```python
from build123d import *

# Parameters (mm, degrees)
SKETCH1_R           = 27.5
BOSS_EXTRUDE1_DEPTH = 30
SKETCH2_R           = 35
BOSS_EXTRUDE2_DEPTH = 20
SKETCH3_R           = 27.5
BOSS_EXTRUDE3_DEPTH = 53
SKETCH4_R           = 5
BOSS_EXTRUDE4_DEPTH = 10
BOSS_EXTRUDE5_START = 50
SKETCH5_R           = 27.5
BOSS_EXTRUDE5_DEPTH = 50
SKETCH8_W           = 100
SKETCH8_H           = 20
BOSS_EXTRUDE6_DEPTH = 30


with BuildPart() as part:
    # Sketch1 → Boss-Extrude1 (new body)
    with BuildSketch(Plane.XY):
        Circle(SKETCH1_R)
    extrude(amount=BOSS_EXTRUDE1_DEPTH)

    # Sketch2 → Boss-Extrude2 (add)
    with BuildSketch(Plane.XY.offset(30)):
        Circle(SKETCH2_R)
    extrude(amount=BOSS_EXTRUDE2_DEPTH)

    # Sketch3 → Boss-Extrude3 (add)
    with BuildSketch(Plane.XY.offset(50)):
        Circle(SKETCH3_R)
    extrude(amount=BOSS_EXTRUDE3_DEPTH)

    # Sketch4 → Boss-Extrude4 (add)
    with BuildSketch(Plane.XY.offset(103)):
        Circle(SKETCH4_R)
    extrude(amount=BOSS_EXTRUDE4_DEPTH)

    # Sketch5 → Boss-Extrude5 (add)
    with BuildSketch(Plane(origin=(0, 0, 0), x_dir=(-1, 0, 0), z_dir=(0, 0, -1)).offset(BOSS_EXTRUDE5_START)):
        Circle(SKETCH5_R)
    extrude(amount=-BOSS_EXTRUDE5_DEPTH)

    # Sketch8 → Boss-Extrude6 (add)
    with BuildSketch(Plane(origin=(0, 0, -50), x_dir=(-1, 0, 0), z_dir=(0, 0, -1))):
        Rectangle(SKETCH8_W, SKETCH8_H)
    extrude(amount=-BOSS_EXTRUDE6_DEPTH)


solid = part.part
```
Can you work these out from the model? Positions are in its coordinate system, mm. A direction names the side the tool comes from. Round coordinates to 2 decimals unless told otherwise and drop trailing zeros. Loops run counter-clockwise (first coordinate to the right, second up) from the corner with the lowest first, then second, coordinate; pieces in that order, holes last. Notation, with made-up numbers: (41, 68) -> (76, 68) arc R12 ccw to (76, 75) -> close; hole circle Ø4 at (56.5, 29). An arc over 180 degrees is marked (long way). Answer in a Markdown table with one row per item.
Item 1: Suppose I cut it at B-B, the plane x = 0. List the corners of the cut face in (y, z) for me, plus the area to 4 significant figures.
Answer block:
| item | result |
|---|---|
| outline | (-35, 30) -> (-27.5, 30) -> (-27.5, -50) -> (27.5, -50) -> (27.5, 30) -> (35, 30) -> (35, 50) -> (27.5, 50) -> (27.5, 103) -> (5, 103) -> (5, 113) -> (-5, 113) -> (-5, 103) -> (-27.5, 103) -> (-27.5, 50) -> (-35, 50) -> close |
| area | 8,815 mm² |
Item 2: Suppose I cut it at D-D, the plane x = -13.5. List the corners of the cut face in (y, z) for me.
Answer block:
| item | result |
|---|---|
| outline | (-32.29, 30) -> (-23.96, 30) -> (-23.96, -50) -> (23.96, -50) -> (23.96, 30) -> (32.29, 30) -> (32.29, 50) -> (23.96, 50) -> (23.96, 103) -> (-23.96, 103) -> (-23.96, 50) -> (-32.29, 50) -> close |
Item 3: If I drill on probe 1 along Z at (x, y) = (-9.5, 10); probe 2 along Z at (x, y) = (-36, 2); probe 3 along Y at (x, z) = (31, -30.5), over which ranges is the centre line in solid material (lowest first)?
Answer block:
| item | result |
|---|---|
| probe 1 | -50 to 103 |
| probe 2 | -50 to -20 |
| probe 3 | -10 to 10 |
Item 4: On a 3-axis mill with a long thin cutter (end or side, diameter ignored), from which of +Z, -Z, +X, -X, +Y, -Y can I reach the whole of each face in a straight line? I mean faces 5 (the flat face through (38, 10, -35)), 6 (the flat face through (-38, -10, -35)), 7 (the flat face through (-38, 10, -35)), 8 (the flat face through (-21, -18, 30)), 9 (the cylindrical face through (-1.08, -4.88, 107.93)). Say none if no direction works.
Answer block:
| item | result |
|---|---|
| face 5 | -Z, +X, +Y |
| face 6 | -Z, -X, -Y |
| face 7 | -Z, -X, +Y |
| face 8 | none |
| face 9 | +Z |
Item 5: Suppose I cut it at C-C, the plane z = 6.5. List the corners of the cut face in (x, y) for me, plus the area to 3 significant figures.
Answer block:
| item | result |
|---|---|
| outline | circle Ø55 at (0, 0) |
| area | 2,380 mm² |
Item 6: We'd pull the mould along Z, two halves only. Please class faces 1 (the flat face through (1, 0, -50)), 2 (the flat face through (38, 0, -20)), 3 (the flat face through (38, -10, -35)), 4 (the flat face through (-38, 0, -20)): released by +Z, released by -Z, zero draft, split by the parting line, or undercut.
Answer block:
| item | result |
|---|---|
| face 1 | released by -Z |
| face 2 | undercut |
| face 3 | zero draft |
| face 4 | undercut |
Item 7: Will these pins go through, and if not, where does the flat tip stop? P1, Ø3, axis at x = 17.5, y = -26.5, coming from the -Z side; P2, Ø7.5, axis at x = 38.5, z = -37, coming from the +Y side; P3, Ø6, axis at y = -6, z = 37.5, coming from the +X side.
Answer block:
| item | result |
|---|---|
| P1 | z = 30 |
| P2 | y = 10 |
| P3 | x = 34.87 |
Item 8: Suppose I cut it at A-A, the plane y = 0. List the corners of the cut face in (x, z) for me, plus the area to 3 significant figures.
Answer block:
| item | result |
|---|---|
| outline | (-50, -50) -> (50, -50) -> (50, -20) -> (27.5, -20) -> (27.5, 30) -> (35, 30) -> (35, 50) -> (27.5, 50) -> (27.5, 103) -> (5, 103) -> (5, 113) -> (-5, 113) -> (-5, 103) -> (-27.5, 103) -> (-27.5, 50) -> (-35, 50) -> (-35, 30) -> (-27.5, 30) -> (-27.5, -20) -> (-50, -20) -> close |
| area | 10,200 mm² |
